```python
from build123d import *

# Parameters (mm, degrees)
F0_R     = 1.5
F1_DEPTH = 3
F3_DEPTH = 1
F5_DEPTH = 0.5


with BuildPart() as f1:
    # F0 (on Top) → F1 (new body)
    with BuildSketch(Plane.XY):
        with BuildLine():
            ThreePointArc((3.4500828672, 21.7277916091), (0, 25.4608047039), (-3.4500828672, 21.7277916091))
            ThreePointArc((-3.4500828672, 21.7277916091), (0, -22), (3.4500828672, 21.7277916091))
        make_face()
        with Locations((0, 22)):
            Circle(F0_R, mode=Mode.SUBTRACT)
    extrude(amount=F1_DEPTH)



with BuildPart() as f3:
    # F2 (on face) → F3 (new body)
    with BuildSketch(Plane.XY.offset(3)):
        Polygon((4.922974389, 6.8000350147), (-4.9908645451, 6.8000350147), (-8.1190178171, -2.440047916), (0, -8.3594759926), (8.0511281267, -2.5844241027), align=None)
    extrude(amount=F3_DEPTH)


with BuildPart() as f3b:
    # F2 (on face) → F3, piece 2 (new body)
    with BuildSketch(Plane.XY.offset(3)):
        with BuildLine():
            ThreePointArc((-1.0919588755, 20.9715906388), (-14.4580228944, -15.2304156901), (20.9999997169, 0))
            ThreePointArc((20.9999997169, 0), (15.2304156901, 14.4580228944), (1.0919588755, 20.9715906388))
            ThreePointArc((1.0919588755, 20.9715906388), (0, 20.5), (-1.0919588755, 20.9715906388))
        make_face()
        with BuildLine():
            ThreePointArc((-16.1295580852, -11.8252846044), (-19.0077768519, -6.2212875796), (-20, 0))
            Line((-20, 0), (-16.4255090058, 0))
            Line((-16.4255090058, 0), (-12.9916435108, 9.2311538756))
            Line((-12.9916435108, 9.2311538756), (-16.1823943196, 11.7528768429))
            ThreePointArc((-16.1823943196, 11.7528768429), (-11.7551151877, 16.1807684281), (-6.1756283357, 19.0226605568))
            Line((-6.1756283357, 19.0226605568), (-4.8075946979, 15.5265759677))
            Line((-4.8075946979, 15.5265759677), (5.26508037, 15.5265759677))
            Line((5.26508037, 15.5265759677), (6.3353531163, 18.9700632812))
            ThreePointArc((6.3353531163, 18.9700632812), (11.7732180825, 16.1676014295), (16.1095758254, 11.8524920048))
            Line((16.1095758254, 11.8524920048), (13.3346663788, 9.6890022978))
            Line((13.3346663788, 9.6890022978), (16.539607197, 0))
            Line((16.539607197, 0), (20, 0))
            ThreePointArc((20, 0), (19.0338940981, -6.1409181287), (16.2289124537, -11.6885585326))
            Line((16.2289124537, -11.6885585326), (13.3346645162, -9.4834174961))
            Line((13.3346645162, -9.4834174961), (5.150616169, -15.3209902346))
            Line((5.150616169, -15.3209902346), (6.1930771205, -19.0169870321))
            ThreePointArc((6.1930771205, -19.0169870321), (0.1603117546, -19.9993574932), (-5.8874264525, -19.1138224792))
            Line((-5.8874264525, -19.1138224792), (-5.0937519409, -15.4926832765))
            Line((-5.0937519409, -15.4926832765), (-13.2777998224, -9.4261867926))
            Line((-13.2777998224, -9.4261867926), (-16.1295580852, -11.8252846044))
        make_face(mode=Mode.SUBTRACT)
    extrude(amount=F3_DEPTH)


with BuildPart() as f1_1:
    add(f1.part)

    add(f3.part)  # F5 merges F3

    add(f3b.part)  # F5 merges F3b
    # F4 (on face) → F5 (join)
    with BuildSketch(Plane.XY.offset(3)):
        Polygon((-3.9732013829, 15.8563796431), (-4.6360646375, 16.1158889532), (-8.0390470102, 11.3176852465), (-13.9602348208, 9.480074048), (-13.2939470932, 8.5717067122), (-8.2003781572, 10.1312547922), (-5.0240522251, 6.0106148012), (-4.1660062867, 6.6720250605), (-7.3132961988, 10.9754130244), align=None)
        Polygon((5.1279528998, 16.2930767983), (4.4984105043, 15.8638432622), (7.6175061986, 11.1995087937), (4.1550239548, 6.6210199147), (4.8672661829, 6.0823867253), (8.3251015592, 10.6547309861), (13.9129273593, 9.0533420444), (14.1338557053, 9.8242410304), (8.3615100011, 11.7145888507), align=None)
        Polygon((13.0210139809, -3.5926375928), (7.2665498592, -1.7012254102), (6.9803940132, -2.7600007597), (12.5604271889, -4.763089586), (12.8751983866, -10.514815338), (14.1574915833, -10.4446400579), (13.8542868014, -4.9042641757), (17.5109170377, 0.5307878018), (16.6018719511, 1.1423811709), align=None)
        Polygon((0.5418943474, -7.1095651947), (-0.6027278141, -7.1095651947), (-0.6027278141, -13.2905244827), (-5.9576934658, -15.2252613613), (-5.6676808745, -16.2379276007), (0.4274321254, -14.4923776388), (5.8904200537, -16.0708622457), (6.1791581102, -15.3508447111), (0.5418943474, -13.0902156234), align=None)
        Polygon((-16.3739044219, 1.1117858812), (-17.4086019397, 0.6545940414), (-13.5853170573, -4.5247467198), (-13.8709158044, -10.2605167986), (-12.7163715661, -10.3180045262), (-12.4276187271, -4.5188898221), (-6.8210065365, -2.7600007597), (-7.3744487017, -1.7012254102), (-12.8848105669, -3.3157542348), align=None)
    extrude(amount=F5_DEPTH)


solid = f1_1.part
```
The listing builds one solid part. Answer for the finished solid, in the listing's coordinates (mm). Round coordinates to 2 decimals unless told otherwise and drop trailing zeros. Write each loop counter-clockwise with the first axis right and the second up, starting at its lowest first coordinate (ties: lowest second). Pieces come first, ordered by that corner, then holes. Notation, with made-up numbers: (55, 73) -> (77, 73) arc R21 ccw to (77, 109) -> close; hole circle Ø7 at (48, -33.75). An arc over 180 degrees is marked (long way). Write item = value, one per line.
1) Section B-B on z = 1.7 is taken. Write down the section's boundary in (x, y).
Check values:
outline = (-3.45, 21.73) arc R22 ccw (long way) to (3.45, 21.73) arc R3.46 ccw (long way) to start; hole circle Ø3 at (0, 22)
2) Straight lines are drawn through the part: line 1 along X through (y, z) = (22, 1.55); line 2 along Z through (x, y) = (9, 0); line 3 along Z through (x, y) = (14, -4). For each, find the intervals that lie inside material, in ascending order. Write a range as [from, to].
Check values:
line_1 = [-3.46, -1.5], [1.5, 3.46]
line_2 = [0, 3]
line_3 = [0, 3.5]
3) Given pin 1 (3.5 mm diameter, centred on x = 0, y = 22, fed in from -Z); pin 2 (6 mm diameter, centred on x = 14, y = -6, fed in from +Z); pin 3 (4.5 mm diameter, centred on x = 11, y = 13.5, fed in from +Z); pin 4 (2 mm diameter, centred on y = 15, z = 0.5, fed in from -X), each flat-ended and moving along its own axis, determine where each tip first touches the part or whether it passes through.
Check values:
pin_1 = 0
pin_2 = 3.5
pin_3 = 3
pin_4 = -16.97
4) Section C-C on y = 3.5 is taken. Write down the section's boundary in (x, z).
Check values:
outline = (-21.72, 0) -> (21.72, 0) -> (21.72, 3) -> (20.71, 3) -> (20.71, 4) -> (15.38, 4) -> (15.38, 3) -> (6.02, 3) -> (6.02, 4) -> (-6.11, 4) -> (-6.11, 3) -> (-15.12, 3) -> (-15.12, 4) -> (-20.71, 4) -> (-20.71, 3) -> (-21.72, 3) -> close
5) Section A-A on y = 13 is taken. Write down the section's boundary in (x, z).
Check values:
outline = (-17.75, 0) -> (17.75, 0) -> (17.75, 3) -> (16.49, 3) -> (16.49, 4) -> (15.2, 4) -> (15.2, 3) -> (7.45, 3) -> (7.45, 3.5) -> (6.41, 3.5) -> (6.41, 3) -> (-5.93, 3) -> (-5.93, 3.5) -> (-6.85, 3.5) -> (-6.85, 3) -> (-15.2, 3) -> (-15.2, 4) -> (-16.49, 4) -> (-16.49, 3) -> (-17.75, 3) -> close
6) Section D-D on y = -6 is taken. Write down the section's boundary in (x, z), plus the area to 3 significant figures.
Check values:
outline = (-21.17, 0) -> (21.17, 0) -> (21.17, 3) -> (20.12, 3) -> (20.12, 4) -> (19.08, 4) -> (19.08, 3) -> (13.91, 3) -> (13.91, 3.5) -> (12.63, 3.5) -> (12.63, 3) -> (3.29, 3) -> (3.29, 4) -> (-3.24, 4) -> (-3.24, 3) -> (-12.5, 3) -> (-12.5, 3.5) -> (-13.66, 3.5) -> (-13.66, 3) -> (-19.08, 3) -> (-19.08, 4) -> (-20.12, 4) -> (-20.12, 3) -> (-21.17, 3) -> close
area = 137 mm²
7) For a pull along X with two mould halves and no side action, classify faces 1 (the cylindrical face through (0.08, 25.46, 1.48)), 2 (the flat face through (-9.13, -12.5, 3.49)) as released by +X, released by -X, zero draft, split by the parting line, or undercut.
Check values:
face_1 = split by the parting line
face_2 = undercut
